Read the model definition and answer for the solid it produces. Units are mm, in the model's axes. A direction names the side the tool comes from. Give positions to 0.01 mm unless a question says otherwise; leave off trailing zeros. Write each loop counter-clockwise with the first axis right and the second up, starting at its lowest first coordinate (ties: lowest second). Pieces come first, ordered by that corner, then holes. Notation, with made-up numbers: M 27.25,-17.5 L 78.25,-17.5 A17 cw 78.25,-13.5 Z; hole C 83.5,36 d4. An arc over 180 degrees is marked long. Write each question's results on one line, items separated by ' | '. Start each with the question number.
```python
from build123d import *

# Parameters (mm, degrees)
BOSS_EXTRUDE2_DEPTH = 10
SKETCH2_R           = 4.25
CUT_EXTRUDE1_DEPTH  = 4.02
SKETCH3_R           = 1.3
CUT_EXTRUDE2_DEPTH  = 56.812278219


with BuildPart() as part:
    # Sketch1 → Boss-Extrude2 (new body)
    with BuildSketch(Plane(origin=(0, 0, 0), x_dir=(1, 0, 0), z_dir=(0, 1, 0))):
        Polygon((0, 0), (0, 29.5), (47, 29.5), (47, 0), (30.5, 0), (30.5, 12.6), (15.5, 12.6), (15.5, 0), align=None)
    extrude(amount=BOSS_EXTRUDE2_DEPTH)

    # Sketch2 → Cut-Extrude1 (cut)
    with BuildSketch(Plane(origin=(0, 10, 0), x_dir=(1, 0, 0), z_dir=(0, 1, 0))):
        with Locations(Location((41.4, 7.45, 0), (0, 0, 270))):
            Circle(SKETCH2_R)
        with Locations(Location((5.6, 7.45, 0), (0, 0, 90))):
            Circle(SKETCH2_R)
        with Locations(Location((5.6, 21.49, 0), (0, 0, 270))):
            Circle(SKETCH2_R)
        with Locations(Location((41.4, 21.49, 0), (0, 0, 90))):
            Circle(SKETCH2_R)
    extrude(amount=-CUT_EXTRUDE1_DEPTH, mode=Mode.SUBTRACT)

    # Sketch3 → Cut-Extrude2 (cut, through all)
    with BuildSketch(Plane(origin=(0, 5.98, 0), x_dir=(1, 0, 0), z_dir=(0, 1, 0))):
        with Locations(Location((5.6, 7.45, 0), (0, 0, 270))):
            Circle(SKETCH3_R)
        with Locations(Location((41.4, 7.45, 0), (0, 0, 270))):
            Circle(SKETCH3_R)
        with Locations(Location((5.6, 21.49, 0), (0, 0, 270))):
            Circle(SKETCH3_R)
        with Locations(Location((41.4, 21.49, 0), (0, 0, 270))):
            Circle(SKETCH3_R)
    extrude(amount=-CUT_EXTRUDE2_DEPTH, mode=Mode.SUBTRACT)


solid = part.part
```
Item 1: For faces 4 (the cylindrical face through (45.55, 8.02, -20.57)), 5 (the cylindrical face through (40.13, 3.03, -21.77)), 6 (the flat face through (15.5, 5, -6)), determine the directions among +Z, -Z, +X, -X, +Y, -Y from which every point of the face is accessible in a straight line to the end or side of a thin tool.
Item 2: Section C-C, the plane y = 3.25 is taken. Determine the outline of the cut face in (x, z), then the cut area to 3 significant figures.
Item 3: Section A-A, the plane z = -21.49 is taken. Determine the outline of the cut face in (x, y).
Item 4: Determine the mould class of faces 1 (the flat face through (23, 5, -12.6)), 2 (the cylindrical face through (3.972, 8.018, -17.564)), 3 (the flat face through (47, 5, -15)) for opening direction Z: +Z half, -Z half, draft (parallel to the pull), parting line (faces both ways), or undercut.
Item 5: Given P1, Ø5, axis at x = 25, y = 6, coming from the +Z side; P2, Ø4, axis at x = 7, z = -20.5, coming from the +Y side, each flat-ended and moving along its own axis, determine where each tip first touches the part or whether it passes through.
Item 6: Section D-D, the plane z = -7.45 is taken. Determine the outline of the cut face in (x, y).
Item 7: Section B-B, the plane x = 5.6 is taken. Determine the outline of the cut face in (y, z).
Item 8: Straight lines are drawn through the part: line 1 (X direction, y = 1.75, z = -21.49); line 2 (X direction, y = 6.95, z = -21.49); line 3 (X direction, y = 4.5, z = -4.5). For each, find the intervals that lie inside material, in ascending order.
Worked out:
1) face 4: +Y | face 5: +Y, -Y | face 6: +Z, +Y, -Y
2) outline: M 0,-29.5 L 47,-29.5 L 47,0 L 30.5,0 L 30.5,-12.6 L 15.5,-12.6 L 15.5,0 L 0,0 Z; hole C 5.6,-21.49 d2.6; hole C 5.6,-7.45 d2.6; hole C 41.4,-21.49 d2.6; hole C 41.4,-7.45 d2.6 | area: 1,180 mm²
3) outline: M 0,0 L 4.3,0 L 4.3,5.98 L 1.35,5.98 L 1.35,10 L 0,10 Z; M 6.9,0 L 40.1,0 L 40.1,5.98 L 37.15,5.98 L 37.15,10 L 9.85,10 L 9.85,5.98 L 6.9,5.98 Z; M 42.7,0 L 47,0 L 47,10 L 45.65,10 L 45.65,5.98 L 42.7,5.98 Z
4) face 1: +Z half | face 2: undercut | face 3: draft
5) P1: stops at z = -12.6 | P2: stops at y = 5.98
6) outline: M 0,0 L 4.3,0 L 4.3,5.98 L 1.35,5.98 L 1.35,10 L 0,10 Z; M 6.9,0 L 15.5,0 L 15.5,10 L 9.85,10 L 9.85,5.98 L 6.9,5.98 Z; M 30.5,0 L 40.1,0 L 40.1,5.98 L 37.15,5.98 L 37.15,10 L 30.5,10 Z; M 42.7,0 L 47,0 L 47,10 L 45.65,10 L 45.65,5.98 L 42.7,5.98 Z
7) outline: M 0,-29.5 L 10,-29.5 L 10,-25.74 L 5.98,-25.74 L 5.98,-22.79 L 0,-22.79 Z; M 0,-20.19 L 5.98,-20.19 L 5.98,-17.24 L 10,-17.24 L 10,-11.7 L 5.98,-11.7 L 5.98,-8.75 L 0,-8.75 Z; M 0,-6.15 L 5.98,-6.15 L 5.98,-3.2 L 10,-3.2 L 10,0 L 0,0 Z
8) line 1: x = 0 to 4.3, 6.9 to 40.1, 42.7 to 47 | line 2: x = 0 to 1.35, 9.85 to 37.15, 45.65 to 47 | line 3: x = 0 to 15.5, 30.5 to 47
